```python
from build123d import *

# Parameters (mm, degrees)
SKETCH1_W               = 100.076
SKETCH1_H               = 228.6
BOSS_EXTRUDE1_DEPTH     = 12.7
SKETCH2_W               = 81.026
SKETCH2_H               = 76.2
CUT_EXTRUDE1_DEPTH      = 13.7
SKETCH3_W               = 20.32
SKETCH3_H               = 41.148
SKETCH3_W_2             = 10.9982
SKETCH3_H_2             = 5.08
CUT_EXTRUDE2_DEPTH      = 13.7
SKETCH4_R               = 3.175
CUT_EXTRUDE3_DEPTH      = 91.551
CUT_EXTRUDE3_DEPTH_BACK = 10.525


with BuildPart() as part:
    # Sketch1 → Boss-Extrude1 (new body)
    with BuildSketch(Plane(origin=(0, 0, 0), x_dir=(1, 0, 0), z_dir=(0, 1, 0))):
        Rectangle(SKETCH1_W, SKETCH1_H)
    extrude(amount=BOSS_EXTRUDE1_DEPTH)

    # Sketch2 → Cut-Extrude1 (cut, through all)
    with BuildSketch(Plane(origin=(0, 12.7, 0), x_dir=(1, 0, 0), z_dir=(0, 1, 0))):
        with Locations((0, -76.2)):
            Rectangle(SKETCH2_W, SKETCH2_H)
    extrude(amount=-CUT_EXTRUDE1_DEPTH, mode=Mode.SUBTRACT)

    # Sketch3 → Cut-Extrude2 (cut, through all)
    with BuildSketch(Plane(origin=(0, 12.7, 0), x_dir=(1, 0, 0), z_dir=(0, 1, 0))):
        with Locations((-30.353, -4.826)):
            Rectangle(SKETCH3_W, SKETCH3_H)
        with Locations((-35.0139, 30.988)):
            Rectangle(SKETCH3_W_2, SKETCH3_H_2)
        with Locations((30.353, -4.826)):
            Rectangle(SKETCH3_W, SKETCH3_H)
        with Locations((35.0139, 30.988)):
            Rectangle(SKETCH3_W_2, SKETCH3_H_2)
    extrude(amount=-CUT_EXTRUDE2_DEPTH, mode=Mode.SUBTRACT)

    # Sketch4 → Cut-Extrude3 (cut, two sides)
    with BuildSketch(Plane(origin=(-40.513, 0, 0), x_dir=(0, 0, -1), z_dir=(1, 0, 0))) as cut_extrude3_sk:
        with Locations((-67.31, 6.35)):
            Circle(SKETCH4_R)
    extrude(amount=CUT_EXTRUDE3_DEPTH, mode=Mode.SUBTRACT)
    extrude(cut_extrude3_sk.sketch, amount=-CUT_EXTRUDE3_DEPTH_BACK, mode=Mode.SUBTRACT)


solid = part.part
```
Geometry: final body of the model. Coordinates: model frame, mm. A direction names the side the tool comes from. Round coordinates to 2 decimals unless told otherwise and drop trailing zeros. Order: outer loops, then holes, each group sorted by start corner. A loop starts at its lowest first (then second) coordinate and runs counter-clockwise, first axis right, second up. Notation, with made-up numbers: M 29.5,73 L 53.5,73 A18 cw 53.5,81 Z; hole C 49,87 d11. An arc over 180 degrees is marked long. One line per item, written item: value.
(1) Cut plane C-C (z = 67.31). Return the cut outline in (x, y) (3 decimals).
Result sheet:
outline: M -50.038,0 L -40.513,0 L -40.513,3.175 L -50.038,3.175 Z; M -50.038,9.525 L -40.513,9.525 L -40.513,12.7 L -50.038,12.7 Z; M 40.513,0 L 50.038,0 L 50.038,3.175 L 40.513,3.175 Z; M 40.513,9.525 L 50.038,9.525 L 50.038,12.7 L 40.513,12.7 Z
(2) Cut plane A-A (y = 6.35). Give the number of separate pieces and of enclosed holes in the cut face, and give its area (3 significant figures).
Result sheet:
separate pieces: 3
enclosed holes: 4
area: 14,800 mm2
(3) Cut plane D-D (z = 7.5). Return the cut outline in (x, y).
Result sheet:
outline: M -50.04,0 L -40.51,0 L -40.51,12.7 L -50.04,12.7 Z; M -20.19,0 L 20.19,0 L 20.19,12.7 L -20.19,12.7 Z; M 40.51,0 L 50.04,0 L 50.04,12.7 L 40.51,12.7 Z
(4) Cut plane B-B (x = 23.5). Return the cut outline in (y, z).
Result sheet:
outline: M 0,-114.3 L 12.7,-114.3 L 12.7,-15.75 L 0,-15.75 Z; M 0,25.4 L 12.7,25.4 L 12.7,38.1 L 0,38.1 Z
(5) Line query: probe 1 along X at (y, z) = (10.5, 11); probe 2 along X at (y, z) = (7.25, -33); probe 3 along Z at (x, y) = (-37.5, 6.25). Output: solid intervals per line, ascending. Write a range as [from, to].
Result sheet:
probe 1: [-50.04, -40.51], [-20.19, 20.19], [40.51, 50.04]
probe 2: [-50.04, -40.51], [-29.51, 29.51], [40.51, 50.04]
probe 3: [-114.3, -33.53], [-28.45, -15.75], [25.4, 38.1]
(6) Reachability of faces 1 (the flat face through (-1, 6, 38.1)), 2 (the flat face through (29.515, 6, -31)), 3 (the flat face through (50.038, 6, 2)) from +Z, -Z, +X, -X, +Y, -Y: full face, straight path, thin tool, end or side. Return the list, or none.
Result sheet:
face 1: +Z, +Y, -Y
face 2: +Y, -Y
face 3: +Z, -Z, +X, +Y, -Y
(7) Pin query (flat end, axial travel): P1, Ø4, axis at x = -30.5, y = 7.5, coming from the +Z side; P2, Ø4, axis at y = 6.35, z = 67.31, coming from the -X side (1 decimal). Return the tip coordinate at first contact, or that it passes through.
Result sheet:
P1: z = 38.1
P2: through
(8) Pull-direction query (Z, two-part tool) for faces 4 (the flat face through (-1, 0, -27)), 5 (the flat face through (-45, 6, 114.3)), 6 (the flat face through (35, 6, -28.448)); classes: pulls with the +Z half, pulls with the -Z half, needs draft (parallel to the pull), parting line crosses it, or undercut.
Result sheet:
face 4: needs draft
face 5: pulls with the +Z half
face 6: undercut
